Read the model definition and answer for the solid it produces. Units are mm, in the model's axes. A direction names the side the tool comes from. Round coordinates to 2 decimals unless told otherwise and drop trailing zeros. Order: outer loops, then holes, each group sorted by start corner. A loop starts at its lowest first (then second) coordinate and runs counter-clockwise, first axis right, second up. Notation, with made-up numbers: (21.5, -12.5) - (70.5, -12.5) arc R29 cw to (70.5, 13.5) - close; hole circle Ø2 at (-6, -12.5). An arc over 180 degrees is marked (long way). Answer as a JSON object with one key per item and string values. Group by question number.
Q1. Given pin 1 Ø6 at (x, y) = (31.5, 9) entering from +Z; pin 2 Ø3 at (y, z) = (18, -166.5) entering from -X; pin 3 Ø6 at (y, z) = (6, 4.5) entering from -X (3 decimals); pin 4 Ø6 at (x, y) = (224.5, 9) entering from -Z, each flat-ended and moving along its own axis, determine where each tip first touches the part or whether it passes through.
Q2. A cutting plane is placed at C-C on y = 9. Determine the outline of the cut face in (x, z) (3 decimals), and give its area (3 significant figures).
Q3. Consider line 1 (Y direction, x = 249, z = -37.5); line 2 (Z direction, x = 272, y = 11); line 3 (X direction, y = 17.75, z = -56). Determine where each line is inside the solid, lowest interval first.
Q4. A cutting plane is placed at D-D on x = 23. Determine the outline of the cut face in (y, z), and give its area (3 significant figures).
Q5. A cutting plane is placed at B-B on x = 244.5. Determine the outline of the cut face in (y, z), and give its area (3 significant figures).
Q6. A tool of negligible diameter and unlimited length cuts with its end or side. For faces 5 (the flat face through (250, 14.288, -62)), 6 (the flat face through (98.425, 10, 4)), 7 (the cylindrical face through (290.791, 10.053, -8.037)), from which of +Z, -Z, +X, -X, +Y, -Y can it reach the whole face along a straight path? Write none if from no direction.
Q7. The mould has two halves that part along X. Classify faces 1 (the cylindrical face through (274.089, 7.044, -60.446)), 2 (the flat face through (18, 10, -188.722)), 3 (the conical face through (298.54, 0.16, -78.72)), 4 (the cylindrical face through (240.675, 17.262, -50.353)): pulls with the +X half, pulls with the -X half, needs draft (parallel to the pull), parting line crosses it, or undercut.
Q8. A cutting plane is placed at A-A on z = -50.8. Determine the outline of the cut face in (x, y) (1 decimal).
```python
from build123d import *

# Parameters (mm, degrees)
F0_R     = 25.1841
F0_R_2   = 10.16
F1_DEPTH = 20.32
F2_DEPTH = 14.2875
F3_DEPTH = 25.4
F4_SIZE  = 2.54


with BuildPart() as f1:
    # F0 (on Front) → F1 (new body)
    with BuildSketch(Plane.XZ):
        with BuildLine():
            Line((98.425, 0), (0, 0))
            Line((0, 0), (0, -188.722))
            Line((0, -188.722), (35.541445, -188.722))
            Line((35.541445, -188.722), (254.477584, -109.443526))
            Line((254.477584, -109.443526), (287.002941, -97.665842))
            ThreePointArc((287.002941, -97.665842), (300.482628, -80.188269), (305.277584, -58.643526))
            Line((305.277584, -58.643526), (305.277584, -43.561))
            ThreePointArc((305.277584, -43.561), (290.398609, -7.639976), (254.477584, 7.239))
            Line((254.477584, 7.239), (152.877584, 7.239))
            Line((152.877584, 7.239), (98.425, 7.239))
            Line((98.425, 7.239), (98.425, 0))
        make_face()
        with Locations((250.825, -50.8)):
            Circle(F0_R, mode=Mode.SUBTRACT)
        with Locations((250.825, -50.8)):
            Circle(F0_R)
        with Locations((250.825, -50.8)):
            Circle(F0_R_2, mode=Mode.SUBTRACT)
        with Locations((250.825, -50.8)):
            Circle(F0_R_2)
    extrude(amount=-F1_DEPTH)

    # F0 (on Front) → F2 (cut)
    with BuildSketch(Plane.XZ):
        with Locations((250.825, -50.8)):
            Circle(F0_R)
        with Locations((250.825, -50.8)):
            Circle(F0_R_2, mode=Mode.SUBTRACT)
    extrude(amount=-F2_DEPTH, mode=Mode.SUBTRACT)

    # F0 (on Front) → F3 (cut)
    with BuildSketch(Plane.XZ):
        with Locations((250.825, -50.8)):
            Circle(F0_R_2)
    extrude(amount=-F3_DEPTH, mode=Mode.SUBTRACT)

    # F4
    f4_edges = [f1.edges().sort_by_distance(p)[0] for p in [
        (176.451292, 0, 7.239),
        (176.451292, 20.32, 7.239),
    ]]
    chamfer(f4_edges, length=F4_SIZE)


solid = f1.part
```
Result set:
{
 "1": {"pin 1": "stops at z = 0", "pin 2": "stops at x = 0", "pin 3": "stops at x = 98.425", "pin 4": "stops at z = -121.38"},
 "2": {"outline": "(0, -188.722) - (35.541, -188.722) - (287.003, -97.666) arc R50.8 ccw to (305.278, -58.644) - (305.278, -43.561) arc R50.8 ccw to (254.478, 7.239) - (98.425, 7.239) - (98.425, 0) - (0, 0) - close; hole circle Ø50.368 at (250.825, -50.8)", "area": "43,200 mm²"},
 "3": {"line 1": "y = 14.29 to 20.32", "line 2": "z = -103.1 to -64.43, -37.17 to 4.12", "line 3": "x = 0 to 242.1, 259.55 to 305.28"},
 "4": {"outline": "(0, -188.72) - (20.32, -188.72) - (20.32, 0) - (0, 0) - close", "area": "3,830 mm²"},
 "5": {"outline": "(0, -113.06) - (20.32, -113.06) - (20.32, -58.75) - (14.29, -58.75) - (14.29, -75.18) - (0, -75.18) - close; (0, -26.42) - (14.29, -26.42) - (14.29, -42.85) - (20.32, -42.85) - (20.32, 4.7) - (17.78, 7.24) - (2.54, 7.24) - (0, 4.7) - close", "area": "1,650 mm²"},
 "6": {"face 5": "-Y", "face 6": "+Z, -X, +Y, -Y", "face 7": "+Z, +X, +Y, -Y"},
 "7": {"face 1": "undercut", "face 2": "needs draft", "face 3": "pulls with the +X half", "face 4": "undercut"},
 "8": {"outline": "(0, 0) - (225.6, 0) - (225.6, 14.3) - (240.7, 14.3) - (240.7, 20.3) - (0, 20.3) - close; (261, 14.3) - (276, 14.3) - (276, 0) - (302.7, 0) - (305.3, 2.5) - (305.3, 17.8) - (302.7, 20.3) - (261, 20.3) - close"}
}
